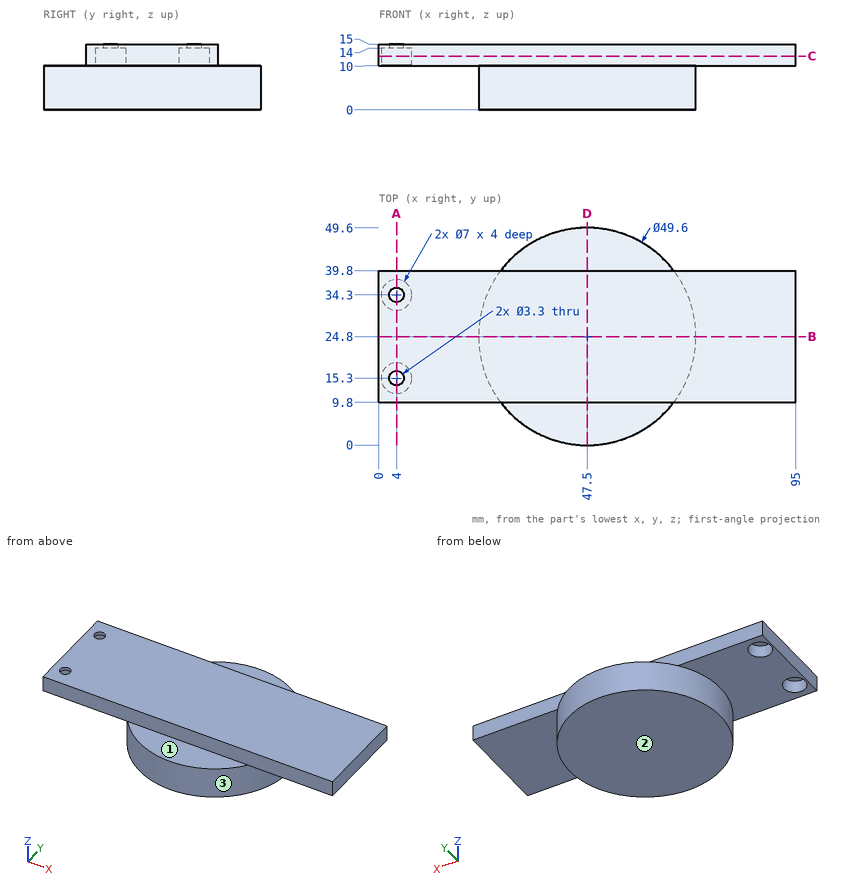
Verification items for this drawing (mm, ordinates from the low corner). A direction names the side the tool comes from. Give positions to 0.01 mm unless a question says otherwise; leave off trailing zeros. Write each loop counter-clockwise with the first axis right and the second up, starting at its lowest first coordinate (ties: lowest second). Pieces come first, ordered by that corner, then holes.
1) Section check B-B, the plane y = 24.8. Record the boundary of the cut face in (x, z).
2) Section check D-D, the plane x = 47.5. Record the boundary of the cut face in (y, z), and give its area (3 significant figures).
3) Gauge pin test, flat ends, axial feed: pin 1 (8 mm diameter, centred on x = 21.5, z = 7, fed in from +Y); pin 2 (5.5 mm diameter, centred on x = 4, y = 34.3, fed in from -Z); pin 3 (8 mm diameter, centred on y = 10, z = 4, fed in from +X). Record the tip position at first contact, or that the pin passes through.
4) Access from +Z, -Z, +X, -X, +Y, -Y to the whole of each face (thin tool, end or side, straight path). Record for the marked faces 1, 2 and 3.
5) Material ranges on L1, parallel to Y at x = 4, z = 14.35; L2, parallel to Y at x = 4, z = 10.8; L3, parallel to X at y = 15.3, z = 14.75, recorded low to high.
6) Section check A-A, the plane x = 4. Record the boundary of the cut face in (y, z), and give its area (3 significant figures).
7) Section check C-C, the plane z = 12.25. Record the boundary of the cut face in (x, y), and give its area (3 significant figures).
Computed:
1. outline: (0, 10) - (22.7, 10) - (22.7, 0) - (72.3, 0) - (72.3, 10) - (95, 10) - (95, 15) - (0, 15) - close
2. outline: (0, 0) - (49.6, 0) - (49.6, 10) - (39.8, 10) - (39.8, 15) - (9.8, 15) - (9.8, 10) - (0, 10) - close
2. area: 646 mm2
3. pin 1: stops at y = 39.8
3. pin 2: stops at z = 14
3. pin 3: stops at x = 69.82
4. face 1: +Z, +X, -X, -Y
4. face 2: -Z, +X, -X, +Y, -Y
4. face 3: -Z
5. L1: y = 9.8 to 13.65, 16.95 to 32.65, 35.95 to 39.8
5. L2: y = 9.8 to 11.8, 18.8 to 30.8, 37.8 to 39.8
5. L3: x = 0 to 2.35, 5.65 to 95
6. outline: (9.8, 10) - (11.8, 10) - (11.8, 14) - (13.65, 14) - (13.65, 15) - (9.8, 15) - close; (16.95, 14) - (18.8, 14) - (18.8, 10) - (30.8, 10) - (30.8, 14) - (32.65, 14) - (32.65, 15) - (16.95, 15) - close; (35.95, 14) - (37.8, 14) - (37.8, 10) - (39.8, 10) - (39.8, 15) - (35.95, 15) - close
6. area: 87.4 mm2
7. outline: (0, 9.8) - (95, 9.8) - (95, 39.8) - (0, 39.8) - close; hole circle Ø7 at (4, 15.3); hole circle Ø7 at (4, 34.3)
7. area: 2,770 mm2
